```python
from build123d import *

# Parameters (mm, degrees)
SKETCH1_R           = 1.7
BOSS_EXTRUDE1_DEPTH = 6


with BuildPart() as part:
    # Sketch1 → Boss-Extrude1 (new body)
    with BuildSketch(Plane(origin=(0, 0, 0), x_dir=(0, 0, -1), z_dir=(1, 0, 0))):
        with BuildLine():
            Line((14.520034317, 1.08101962), (-6.126384754, -6.516702375))
            ThreePointArc((-6.126384754, -6.516702375), (-11.26168313, -4.144211997), (-8.889192752, 0.991086378))
            Line((-8.889192752, 0.991086378), (11.757226319, 8.588808374))
            ThreePointArc((11.757226319, 8.588808374), (16.892524695, 6.216317996), (14.520034317, 1.08101962))
        make_face()
        Circle(SKETCH1_R, mode=Mode.SUBTRACT)
        with Locations((-7.507788753, -2.762807998)):
            Circle(SKETCH1_R, mode=Mode.SUBTRACT)
    extrude(amount=-BOSS_EXTRUDE1_DEPTH)


solid = part.part
```
Source: CAD feature listing. Evaluate the final solid. Frame: model axes, mm. Coordinates: 2 decimals unless noted, no trailing zeros. Loops run counter-clockwise (first coordinate to the right, second up) from the corner with the lowest first, then second, coordinate; pieces in that order, holes last. Notation, with made-up numbers: M -18.75,43.25 L -3.75,43.25 A11 cw -3.75,50.25 Z; hole C 63.5,0 d2. An arc over 180 degrees is marked long. Put each result on its own line as item: value. Start each with the question number.
1) Cut plane B-B on y = 0. Return the cut outline in (x, z), then the cut area to 3 significant figures.
2) Cut plane C-C on x = -5.15. Return the cut outline in (y, z).
3) Ray query, L1, parallel to Y at x = -3.25, z = 7.75; L2, parallel to Y at x = -4.35, z = 0; L3, parallel to Y at x = -2.45, z = -4.5. Return the intervals inside material, ascending. Write a range as from..to.
4) Cut plane A-A on z = 0. Return the cut outline in (x, y).
5) Contact query for flat-ended pins moving along their axis: pin 1 Ø3 at (y, z) = (-2.76, 7.51) entering from +X; pin 2 Ø3 at (x, z) = (-4.5, -9) entering from -Y. Output: stop coordinate, or through.
6) Pull-direction query (Y, two-part tool) for faces 1 (the face through (-2.96, -1.66, 0.37)), 2 (the face through (-2.958, -2.665, -4.341)), 3 (the face through (-2.958, 4.737, -1.289)); classes: pulls with the +Y half, pulls with the -Y half, needs draft (parallel to the pull), parting line crosses it, or undercut.
7) Cut plane D-D on y = 2.5. Return the cut outline in (x, z), then the cut area to 3 significant figures.
The answers:
1. outline: M -6,-11.58 L 0,-11.58 L 0,-1.7 L -6,-1.7 Z; M -6,1.7 L 0,1.7 L 0,10.4 L -6,10.4 Z
1. area: 111 mm²
2. outline: M -6.52,6.13 L 1.08,-14.52 A4 ccw 8.59,-11.76 L 0.99,8.89 A4 ccw Z; hole C -2.76,7.51 d3.4; hole C 0,0 d3.4
3. L1: y = -6.76..-4.45, -1.08..1.41
3. L2: y = -4.26..-1.7, 1.7..4.26
3. L3: y = -2.61..5.92
4. outline: M -6,-4.26 L 0,-4.26 L 0,-1.7 L -6,-1.7 Z; M -6,1.7 L 0,1.7 L 0,4.26 L -6,4.26 Z
5. pin 1: passes through
5. pin 2: stops at y = -1.5
6. face 1: undercut
6. face 2: pulls with the -Y half
6. face 3: pulls with the +Y half
7. outline: M -6,-16.39 L 0,-16.39 L 0,4.79 L -6,4.79 Z
7. area: 127 mm²
